Geometry check sheet. Reference: drawing and pictorial views, mm from the part's lowest x, y, z. A direction names the side the tool comes from. Give positions to 0.01 mm unless a question says otherwise; leave off trailing zeros. Order: outer loops, then holes, each group sorted by start corner. A loop starts at its lowest first (then second) coordinate and runs counter-clockwise, first axis right, second up. Notation, with made-up numbers: (-27, 12) - (-12, 12) arc R24 cw to (-12, 29) - close; hole circle Ø9 at (20, 28.25). An arc over 180 degrees is marked (long way). Answer as a JSON object with one key per item and string values.
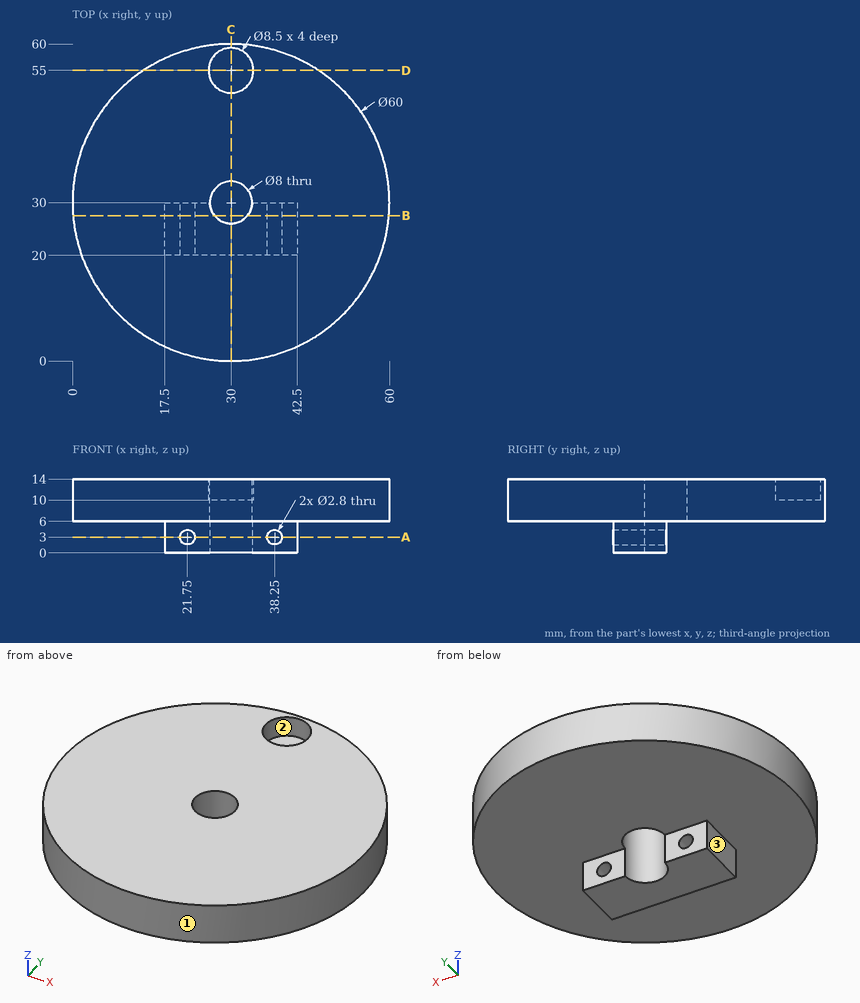
(1) Access from +Z, -Z, +X, -X, +Y, -Y to the whole of each face (thin tool, end or side, straight path). Record for the marked faces 1, 2 and 3.
Computed values:
{"face 1": "+Z, -Z", "face 2": "+Z", "face 3": "-Z, -X, +Y, -Y"}
(2) Section check C-C (x = 30). Record the cut outline in (y, z).
Computed values:
{"outline": "(0, 6) - (20, 6) - (20, 0) - (26, 0) - (26, 14) - (0, 14) - close; (34, 6) - (60, 6) - (60, 14) - (59.25, 14) - (59.25, 10) - (50.75, 10) - (50.75, 14) - (34, 14) - close"}
(3) Section check A-A (z = 3). Record the cut outline in (x, y), then the cut area to 3 significant figures.
Computed values:
{"outline": "(17.5, 20) - (20.35, 20) - (20.35, 30) - (17.5, 30) - close; (23.15, 20) - (36.85, 20) - (36.85, 30) - (34, 30) arc R4 cw to (26, 30) - (23.15, 30) - close; (39.65, 20) - (42.5, 20) - (42.5, 30) - (39.65, 30) - close", "area": "169 mm²"}
(4) Gauge pin test, flat ends, axial feed: pin 1 Ø3 at (y, z) = (22.5, 3) entering from -X; pin 2 Ø2 at (x, z) = (41.5, 7.5) entering from -Y; pin 3 Ø6.5 at (x, z) = (26.5, 3.5) entering from -Y; pin 4 Ø2.5 at (x, z) = (21.75, 3) entering from -Y. Record the tip position at first contact, or that the pin passes through.
Computed values:
{"pin 1": "stops at x = 17.5", "pin 2": "stops at y = 1.9", "pin 3": "stops at y = 0.03", "pin 4": "passes through"}
(5) Section check D-D (y = 55). Record the cut outline in (x, z), then the cut area to 3 significant figures.
Computed values:
{"outline": "(13.42, 6) - (46.58, 6) - (46.58, 14) - (34.25, 14) - (34.25, 10) - (25.75, 10) - (25.75, 14) - (13.42, 14) - close", "area": "231 mm²"}
(6) Material ranges on line 1 along X through (y, z) = (23.25, 3); line 2 along Y through (x, z) = (30, 11); line 3 along Z through (x, y) = (38.25, 26.75), recorded low to high. Write a range as [from, to].
Computed values:
{"line 1": "x = [17.5, 20.35], [23.15, 36.85], [39.65, 42.5]", "line 2": "y = [0, 26], [34, 50.75], [59.25, 60]", "line 3": "z = [0, 1.6], [4.4, 14]"}
(7) Section check B-B (y = 27.5). Record the cut outline in (x, z), then the cut area to 3 significant figures.
Computed values:
{"outline": "(0.1, 6) - (17.5, 6) - (17.5, 0) - (26.88, 0) - (26.88, 14) - (0.1, 14) - close; (33.12, 0) - (42.5, 0) - (42.5, 6) - (59.9, 6) - (59.9, 14) - (33.12, 14) - close; hole circle Ø2.8 at (21.75, 3); hole circle Ø2.8 at (38.25, 3)", "area": "529 mm²"}
